Work out the finished part from the listing and answer in its coordinate system (mm). Face numbers are marked on the shaded views. Round coordinates to 2 decimals unless told otherwise and drop trailing zeros. Order: outer loops, then holes, each group sorted by start corner. A loop starts at its lowest first (then second) coordinate and runs counter-clockwise, first axis right, second up. Notation, with made-up numbers: (51, -33.5) -> (100, -33.5) arc R16 ccw to (100, -15.5) -> close; hole circle Ø5 at (49, -22.5). An arc over 180 degrees is marked (long way). Use a Markdown table: item, result. Add a question column.
Item 1: A cutting plane is placed at B-B, the plane z = 4.25. Give the number of separate pieces and of enclosed holes in the cut face, plus the area to 3 significant figures.
Item 2: A cutting plane is placed at A-A, the plane y = 27.75. Determine the outline of the cut face in (x, z).
Item 3: For a pull along X with two mould halves and no side action, classify the marked faces 1, 2 and 3 as +X half, -X half, draft (parallel to the pull), parting line (faces both ways), or undercut.
Item 4: Find the intervals of material crossed by L1, parallel to X at y = 29.5, z = 1; L2, parallel to X at y = 27, z = 2.5; L3, parallel to X at y = 29.75, z = 1, in increasing order. Write a range as [from, to].
Item 5: Flat-ended cylindrical pins translate along their axes: P1, Ø1.5, axis at y = 27.5, z = 2.5, coming from the +X side; P2, Ø3, axis at x = -63.5, z = 2.5, coming from the +Y side; P3, Ø1.5, axis at y = 32, z = 3, coming from the +X side. Find the tip coordinate at first contact, or state that the pin passes through.
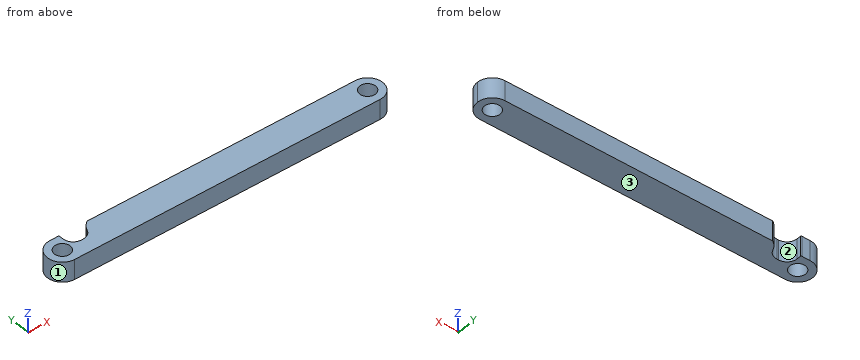
from build123d import *

# Parameters (mm, degrees)
SKETCH1_R           = 2.50825
BOSS_EXTRUDE1_DEPTH = 6.35


with BuildPart() as part:
    # Sketch1 → Boss-Extrude1 (new body)
    with BuildSketch(Plane.XY):
        with BuildLine():
            Line((-62.098423071, 33.11819072), (-62.098423071, 31.791851336))
            ThreePointArc((-62.098423071, 31.791851336), (-61.168487101, 29.546787305), (-58.923423071, 28.616851336))
            Line((-58.923423071, 28.616851336), (-58.325690241, 28.616851336))
            ThreePointArc((-58.325690241, 28.616851336), (-56.534748704, 29.17018137), (-55.368047634, 30.637305881))
            ThreePointArc((-55.368047634, 30.637305881), (-54.438487204, 32.200247817), (-53.054079396, 33.379351336))
            Line((-53.054079396, 33.379351336), (32.357826929, 33.379351336))
            ThreePointArc((32.357826929, 33.379351336), (35.725422975, 31.984447381), (37.120326929, 28.616851336))
            ThreePointArc((37.120326929, 28.616851336), (35.725422975, 25.24925529), (32.357826929, 23.854351336))
            Line((32.357826929, 23.854351336), (-64.964369517, 23.854351336))
            ThreePointArc((-64.964369517, 23.854351336), (-69.723087501, 28.61306932), (-64.964369517, 33.371787305))
            Line((-64.964369517, 33.371787305), (-62.36673293, 33.371787305))
            ThreePointArc((-62.36673293, 33.371787305), (-62.177950586, 33.302785823), (-62.098423071, 33.11819072))
        make_face()
        with Locations((32.357826929, 28.616851336)):
            Circle(SKETCH1_R, mode=Mode.SUBTRACT)
        with Locations((-64.964369517, 28.61306932)):
            Circle(SKETCH1_R, mode=Mode.SUBTRACT)
    extrude(amount=BOSS_EXTRUDE1_DEPTH)


solid = part.part
Reported:
| question | item | result |
|---|---|---|
| 1 | separate pieces | 1 |
| 1 | enclosed holes | 2 |
| 1 | area | 928 mm² |
| 2 | outline | (-69.64, 0) -> (-67.32, 0) -> (-67.32, 6.35) -> (-69.64, 6.35) -> close; (-62.61, 0) -> (30, 0) -> (30, 6.35) -> (-62.61, 6.35) -> close; (34.71, 0) -> (37.04, 0) -> (37.04, 6.35) -> (34.71, 6.35) -> close |
| 3 | face 1 | -X half |
| 3 | face 2 | undercut |
| 3 | face 3 | draft |
| 4 | L1 | [-69.64, -67.31], [-62.62, -61.12], [-56.13, 30.01], [34.71, 37.04] |
| 4 | L2 | [-69.44, -66.89], [-63.04, 30.44], [34.28, 36.84] |
| 4 | L3 | [-69.59, -67.2], [-62.73, -61.35], [-55.89, 30.12], [34.6, 36.98] |
| 5 | P1 | x = 37.11 |
| 5 | P2 | y = 33.37 |
| 5 | P3 | x = 36.33 |
